Geometry: final body of the model. Coordinates: model frame, mm. A direction names the side the tool comes from. Give positions to 0.01 mm unless a question says otherwise; leave off trailing zeros. Write each loop counter-clockwise with the first axis right and the second up, starting at its lowest first coordinate (ties: lowest second). Pieces come first, ordered by that corner, then holes. Notation, with made-up numbers: (-39.75, 52.25) - (-5.75, 52.25) arc R15 cw to (-5.75, 69.25) - close; hole circle Ø4 at (61.25, 1). An arc over 180 degrees is marked (long way). One line per question, with ' | ' between items. Start each with the question number.
```python
from build123d import *

# Parameters (mm, degrees)
CROQUIS1_W                 = 21
CROQUIS1_H                 = 25
SALIENTE_EXTRUIR1_DEPTH    = 20
CROQUIS2_W                 = 21
CROQUIS2_H                 = 25
SALIENTE_EXTRUIR2_DEPTH    = 20
CORTAR_EXTRUIR1_REACH      = 49.746
CROQUIS3_W                 = 12
CROQUIS3_H                 = 6.5
CROQUIS5_R                 = 3.5
CROQUIS5_W                 = 9.5
CROQUIS5_H                 = 3.5
CORTAR_EXTRUIR3_DEPTH      = 25
CROQUIS6_R                 = 4.65
CORTAR_EXTRUIR4_DEPTH      = 3
CORTAR_EXTRUIR5_REACH      = 49.266
CORTAR_EXTRUIR5_END_RADIUS = 3.5
CROQUIS7_R                 = 2.5
REDONDEO4_R                = 4
CROQUIS8_R                 = 3.25
CORTAR_EXTRUIR6_DEPTH      = 9.5
REDONDEO5_R                = 4


with BuildPart() as part:
    # Croquis1 → Saliente-Extruir1 (new body)
    with BuildSketch(Plane(origin=(0, 0, 0), x_dir=(1, 0, 0), z_dir=(0, 1, 0))):
        with Locations((1.75, -2.95)):
            Rectangle(CROQUIS1_W, CROQUIS1_H)
    extrude(amount=SALIENTE_EXTRUIR1_DEPTH)

    # Croquis2 → Saliente-Extruir2 (add)
    with BuildSketch(Plane(origin=(0, 20, 0), x_dir=(1, 0, 0), z_dir=(0, 1, 0))):
        with Locations((1.75, -2.95)):
            Rectangle(CROQUIS2_W, CROQUIS2_H)
    extrude(amount=SALIENTE_EXTRUIR2_DEPTH)

    # Croquis3 → Cortar-Extruir1 (cut, up to next)
    with BuildSketch(Plane.ZY.offset(8.75), mode=Mode.PRIVATE) as cortar_extruir1_sk1:
        with Locations((2.95, 30.25)):
            Rectangle(CROQUIS3_W, CROQUIS3_H)
    cortar_extruir1_tool1 = extrude(cortar_extruir1_sk1.sketch, amount=-CORTAR_EXTRUIR1_REACH, mode=Mode.PRIVATE) & part.part
    add(cortar_extruir1_tool1.solids().sort_by_distance((-8.75, 30.25, 2.95))[0], mode=Mode.SUBTRACT)

    # Croquis5 → Cortar-Extruir3 (cut)
    with BuildSketch(Plane.XZ):
        with Locations(Location((1.75, 0.45, 0), (0, 0, 270))):
            Circle(CROQUIS5_R)
        with Locations((1.75, 6.7)):
            Rectangle(CROQUIS5_W, CROQUIS5_H)
    extrude(amount=-CORTAR_EXTRUIR3_DEPTH, mode=Mode.SUBTRACT)

    # Croquis6 → Cortar-Extruir4 (cut)
    with BuildSketch(Plane.XY.offset(15.45)):
        with Locations((1.75, 7)):
            Circle(CROQUIS6_R)
        with Locations((1.75, 20)):
            Circle(CROQUIS6_R)
    extrude(amount=-CORTAR_EXTRUIR4_DEPTH, mode=Mode.SUBTRACT)

    # Cortar-Extruir5: up to this cylinder (the profile starts outside it)
    cortar_extruir5_end = Plane(origin=(1.75, 13.5, 0.45), z_dir=(0, -1, 0)) * Cylinder(CORTAR_EXTRUIR5_END_RADIUS, 119.532, mode=Mode.PRIVATE)
    # Croquis7 → Cortar-Extruir5 (cut, up to the surface)
    with BuildSketch(Plane.XY.offset(12.45), mode=Mode.PRIVATE) as cortar_extruir5_sk1:
        with Locations((1.75, 20)):
            Circle(CROQUIS7_R)
    cortar_extruir5_tool1 = extrude(cortar_extruir5_sk1.sketch, amount=-CORTAR_EXTRUIR5_REACH, mode=Mode.PRIVATE) - cortar_extruir5_end
    add(cortar_extruir5_tool1.solids().sort_by_distance((1.75, 20, 12.45))[0], mode=Mode.SUBTRACT)
    # Croquis7 → Cortar-Extruir5 (cut, up to the surface)
    with BuildSketch(Plane.XY.offset(12.45), mode=Mode.PRIVATE) as cortar_extruir5_sk2:
        with Locations((1.75, 7)):
            Circle(CROQUIS7_R)
    cortar_extruir5_tool2 = extrude(cortar_extruir5_sk2.sketch, amount=-CORTAR_EXTRUIR5_REACH, mode=Mode.PRIVATE) - cortar_extruir5_end
    add(cortar_extruir5_tool2.solids().sort_by_distance((1.75, 7, 12.45))[0], mode=Mode.SUBTRACT)

    # Redondeo4
    redondeo4_edges = [part.edges().sort_by_distance(p)[0] for p in [
        (12.25, 0, 2.95),
        (-8.75, 0, 2.95),
    ]]
    fillet(redondeo4_edges, radius=REDONDEO4_R)

    # Croquis8 → Cortar-Extruir6 (cut, symmetric)
    with BuildSketch(Plane.XZ.offset(-33.5)):
        with Locations(Location((1.75, 2.95, 0), (0, 0, 270))):
            Circle(CROQUIS8_R)
    extrude(amount=CORTAR_EXTRUIR6_DEPTH, both=True, mode=Mode.SUBTRACT)

    # Redondeo5
    redondeo5_edges = [part.edges().sort_by_distance(p)[0] for p in [
        (1.75, 40, 15.45),
        (12.25, 40, 2.95),
        (1.75, 40, -9.55),
        (-8.75, 40, 2.95),
    ]]
    fillet(redondeo5_edges, radius=REDONDEO5_R)


solid = part.part
```
1) First-contact query: pin 1 Ø6.5 at (x, y) = (1.75, 20) entering from +Z; pin 2 Ø2.5 at (x, z) = (1, 0.5) entering from -Y; pin 3 Ø3.5 at (x, z) = (1, 4) entering from +Y. Flat tips, straight axial feed; report the tip coordinate or a pass-through.
2) Section B-B, the plane x = 7. Output: boundary loops of the cut face in (y, z), plus the area to 3 significant figures.
3) Reachability of faces 4 (the flat face through (-1, 27, 0)), 5 (the cylindrical face through (4.25, 10.92, 13.97)), 6 (the flat face through (2, 12, 8.45)), 7 (the flat face through (1.8, 24, 4.2)) from +Z, -Z, +X, -X, +Y, -Y: full face, straight path, thin tool, end or side. Return the list, or none.
4) Section D-D, the plane z = 4.5. Output: boundary loops of the cut face in (x, y), plus the area to 3 significant figures.
5) Section C-C, the plane z = 10.25. Output: boundary loops of the cut face in (x, y).
6) Line query: L1, parallel to Y at x = 1.75, z = 11; L2, parallel to Y at x = 1.75, z = 4.5; L3, parallel to Z at x = 2, y = 2. Output: solid intervals per line, ascending.
7) Pull-direction query (Z, two-part tool) for faces 1 (the cylindrical face through (1.42, 22.48, 10.48)), 2 (the cylindrical face through (2.8, 12.32, -2.89)), 3 (the flat face through (4, 5, 12.45)); classes: +Z half, -Z half, draft (parallel to the pull), parting line (faces both ways), or undercut.
8) Section A-A, the plane y = 33. Output: boundary loops of the cut face in (x, z).
Answer key:
1) pin 1: z = 12.45 | pin 2: y = 25 | pin 3: y = 24
2) outline: (0, -9.55) - (36, -9.55) arc R4 ccw to (40, -5.55) - (40, 11.45) arc R4 ccw to (36, 15.45) - (0, 15.45) - close; hole (27, -3.05) - (33.5, -3.05) - (33.5, 8.95) - (27, 8.95) - close | area: 915 mm^2
3) face 4: +X, -X | face 5: +Z | face 6: -Y | face 7: +Y
4) outline: (-8.75, 4) arc R4 ccw to (-4.75, 0) - (8.25, 0) arc R4 ccw to (12.25, 4) - (12.25, 27) - (4.61, 27) - (4.61, 24) - (-1.11, 24) - (-1.11, 27) - (-8.75, 27) - close; (-8.75, 33.5) - (-1.11, 33.5) - (-1.11, 40) - (-4.75, 40) arc R4 ccw to (-8.75, 36) - close; (4.61, 33.5) - (12.25, 33.5) - (12.25, 36) arc R4 ccw to (8.25, 40) - (4.61, 40) - close; hole circle Ø5 at (1.75, 7); hole circle Ø5 at (1.75, 20) | area: 596 mm^2
5) outline: (-8.75, 4) arc R4 ccw to (-4.75, 0) - (8.25, 0) arc R4 ccw to (12.25, 4) - (12.25, 36) arc R4 ccw to (8.25, 40) - (-4.75, 40) arc R4 ccw to (-8.75, 36) - close; hole circle Ø5 at (1.75, 7); hole circle Ø5 at (1.75, 20)
6) L1: 0 to 4.5, 9.5 to 17.5, 22.5 to 40 | L2: 0 to 4.5, 9.5 to 17.5, 22.5 to 24 | L3: -9.55 to -3.04, 3.94 to 4.95, 8.45 to 15.45
7) face 1: draft | face 2: undercut | face 3: +Z half
8) outline: (-8.75, -9.55) - (12.25, -9.55) - (12.25, -3.05) - (-8.75, -3.05) - close; (-8.75, 8.95) - (12.25, 8.95) - (12.25, 15.45) - (-8.75, 15.45) - close
